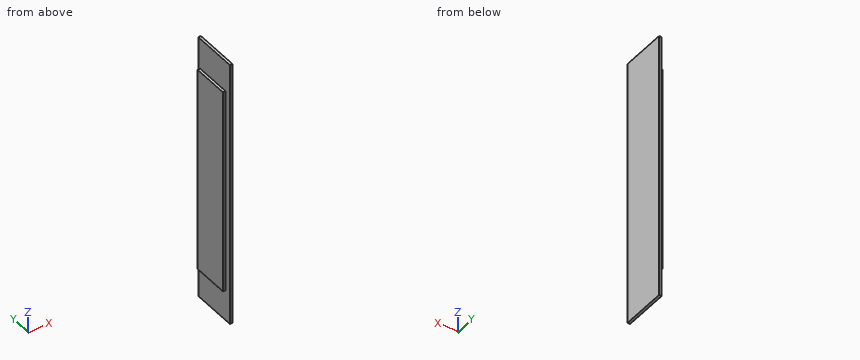
```python
from build123d import *

# Parameters (mm, degrees)
SKETCH1_W           = 35
SKETCH1_H           = 200
BOSS_EXTRUDE1_DEPTH = 2.5
SKETCH2_W           = 260
SKETCH2_H           = 43.5
BOSS_EXTRUDE2_DEPTH = 2.5


with BuildPart() as part:
    # Sketch1 → Boss-Extrude1 (new body, symmetric)
    with BuildSketch(Plane.YZ):
        with Locations((-17.5, 0)):
            Rectangle(SKETCH1_W, SKETCH1_H)
    extrude(amount=BOSS_EXTRUDE1_DEPTH, both=True)

    # Sketch2 → Boss-Extrude2 (add)
    with BuildSketch(Plane(origin=(0, 0, 0), x_dir=(0, 0, -1), z_dir=(1, 0, 0))):
        with Locations((0, -19.25)):
            Rectangle(SKETCH2_W, SKETCH2_H)
    extrude(amount=BOSS_EXTRUDE2_DEPTH)


solid = part.part
```
Build history of the part. All positions in model axes, mm. Round coordinates to 2 decimals unless told otherwise and drop trailing zeros. Loops run counter-clockwise (first coordinate to the right, second up) from the corner with the lowest first, then second, coordinate; pieces in that order, holes last. Notation, with made-up numbers: M 35,57 L 47,57 A25 ccw 47,77 Z; hole C -37,-28.75 d6. An arc over 180 degrees is marked long. Answer as CSV lines item,"result".
1. Cut at C-C on x = -1.75. Write the cut outline in (y, z), then the cut area to 3 significant figures.
Resolved:
outline,"M -35,-100 L 0,-100 L 0,100 L -35,100 Z"
area,"7,000 mm²"
2. Flat gauge pins, fed straight in: P1, Ø1.5, axis at x = -1.5, y = -12.5, coming from the +Z side; P2, Ø1.2, axis at x = -1.5, z = 5.5, coming from the +Y side; P3, Ø1.2, axis at x = -1.5, z = -34, coming from the -Y side. Where does each tip first touch, or does it go through?
Resolved:
P1,"stops at z = 100"
P2,"stops at y = 0"
P3,"stops at y = -35"
3. Wall check: probe 1 along X at (y, z) = (-34.5, -102); probe 2 along Z at (x, y) = (-1.4, -18.5); probe 3 along Y at (x, z) = (-1.2, 79). Give the ranges that are in metal, low to high. Write a range as [from, to].
Resolved:
probe 1,"x = [0, 2.5]"
probe 2,"z = [-100, 100]"
probe 3,"y = [-35, 0]"
4. Cut at B-B on z = -82. Write the cut outline in (x, y).
Resolved:
outline,"M -2.5,-35 L 0,-35 L 0,-41 L 2.5,-41 L 2.5,2.5 L 0,2.5 L 0,0 L -2.5,0 Z"
5. Cut at A-A on y = -22. Write the cut outline in (x, z), then the cut area to 3 significant figures.
Resolved:
outline,"M -2.5,-100 L 0,-100 L 0,-130 L 2.5,-130 L 2.5,130 L 0,130 L 0,100 L -2.5,100 Z"
area,"1,150 mm²"
